```python
from build123d import *

# Parameters (mm, degrees)
F1_DEPTH = 6.35
F2_R     = 7.9375
F3_DEPTH = 76.2
F4_R     = 7.9375
F5_DEPTH = 6.35


with BuildPart() as f1:
    # F0 (on Front) → F1 (new body)
    with BuildSketch(Plane.XZ):
        Polygon((12.464992, 0), (6.232496, 10.795), (-6.232496, 10.795), (-12.464992, 0), (-6.232496, -10.795), (6.232496, -10.795), align=None)
    extrude(amount=F1_DEPTH)

    # F2 (on face) → F3 (join)
    with BuildSketch(Plane(origin=(0, 0, 0), x_dir=(-1, 0, 0), z_dir=(0, 1, 0))):
        Circle(F2_R)
    extrude(amount=F3_DEPTH)

    # F4 (on face) → F5 (join)
    with BuildSketch(Plane(origin=(0, 76.2, 0), x_dir=(-1, 0, 0), z_dir=(0, 1, 0))):
        Polygon((12.464992, 0), (6.232496, 10.795), (-6.232496, 10.795), (-12.464992, 0), (-6.232496, -10.795), (6.232496, -10.795), align=None)
        Circle(F4_R, mode=Mode.SUBTRACT)
        Circle(F4_R)
    extrude(amount=F5_DEPTH)


solid = f1.part
```
Check sheet for the modelled part. Datum: model origin and axes. Units: mm. A direction names the side the tool comes from. Round coordinates to 2 decimals unless told otherwise and drop trailing zeros. Loops run counter-clockwise (first coordinate to the right, second up) from the corner with the lowest first, then second, coordinate; pieces in that order, holes last. Notation, with made-up numbers: (72.25, -29) - (96.25, -29) arc R6 cw to (96.25, -24) - close; hole circle Ø6 at (52, 64.25). An arc over 180 degrees is marked (long way). Answer as a JSON object with one key per item and string values. Group by question number.
Q1. Set-up check for faces 1 (the face through (0, -6.35, 0)), 2 (the face through (8.1, 0, 0.2)): record each of +Z, -Z, +X, -X, +Y, -Y from which the full face is reachable in a straight line by a thin tool's end or side.
Q2. Gauge pin test, flat ends, axial feed: P1, Ø8, axis at x = -5.5, y = 37.5, coming from the -Z side; P2, Ø3, axis at x = -1.5, y = 69, coming from the -Z side; P3, Ø4, axis at y = 37.5, z = 1, coming from the -X side. Record the tip position at first contact, or that the pin passes through.
Q3. Sectioned sample at A-A, the plane x = 9.25. Enter the section's corners in (y, z), plus the area to 3 significant figures.
Q4. Scan lines: line 1 along Y through (x, z) = (-2, 8); line 2 along Z through (x, y) = (-1.25, 26). Record each from-to range of solid material in increasing order. Write a range as [from, to].
Q5. Sectioned sample at B-B, the plane z = 6. Enter the section's corners in (x, y).
Q6. Mould release check, pull along Y, two halves, no side actions. Record for faces 3 (the face through (0, 82.55, 0)), 4 (the face through (-9.305, 79.331, -5.473)), 5 (the face through (-8.1, 76.2, 0.2)): released by +Y, released by -Y, zero draft, split by the parting line, or undercut.
Q7. Sectioned sample at D-D, the plane y = 5. Enter the section's corners in (x, z) (1 decimal).
Solution:
{
 "1": {"face 1": "+Z, -Z, +X, -X, -Y", "face 2": "none"},
 "2": {"P1": "stops at z = -7.79", "P2": "stops at z = -7.94", "P3": "stops at x = -7.94"},
 "3": {"outline": "(-6.35, -5.57) - (0, -5.57) - (0, 5.57) - (-6.35, 5.57) - close; (76.2, -5.57) - (82.55, -5.57) - (82.55, 5.57) - (76.2, 5.57) - close", "area": "141 mm²"},
 "4": {"line 1": "y = [-6.35, 0], [76.2, 82.55]", "line 2": "z = [-7.84, 7.84]"},
 "5": {"outline": "(-9, -6.35) - (9, -6.35) - (9, 0) - (5.2, 0) - (5.2, 76.2) - (9, 76.2) - (9, 82.55) - (-9, 82.55) - (-9, 76.2) - (-5.2, 76.2) - (-5.2, 0) - (-9, 0) - close"},
 "6": {"face 3": "released by +Y", "face 4": "zero draft", "face 5": "undercut"},
 "7": {"outline": "circle Ø15.9 at (0, 0)"}
}
